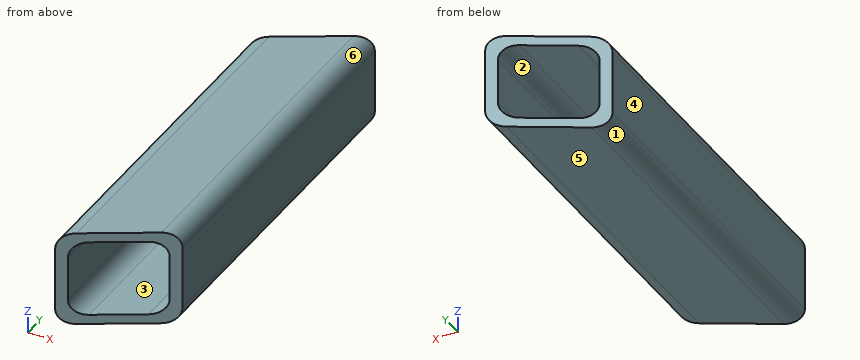
from build123d import *

# Parameters (mm, degrees)
F0_W     = 60
F0_H     = 60
F1_DEPTH = 250
F2_T     = -6
F3_R     = 10
F5_DEPTH = 60.001
F7_DEPTH = 60.001


with BuildPart() as f1:
    # F0 (on Front) → F1 (new body)
    with BuildSketch(Plane.XZ):
        Rectangle(F0_W, F0_H)
    extrude(amount=F1_DEPTH)

    # F2
    f2_openings = [f1.faces().sort_by_distance(p)[0] for p in [
        (0, -250, 0),
        (0, 0, 0),
    ]]
    offset(amount=F2_T, openings=f2_openings)

    # F3
    f3_edges = [f1.edges().sort_by_distance(p)[0] for p in [
        (-30, -125, 30),
        (-24, -125, -24),
        (30, -125, 30),
        (30, -125, -30),
        (-24, -125, 24),
        (-30, -125, -30),
        (24, -125, 24),
        (24, -125, -24),
    ]]
    fillet(f3_edges, radius=F3_R)

    # F4 (on face) → F5 (cut, through all)
    with BuildSketch(Plane.XY.offset(30)):
        Polygon((40, -255.7735026919), (40, -209.5854811567), (-40, -255.7735026919), align=None)
    extrude(amount=-F5_DEPTH, mode=Mode.SUBTRACT)

    # F6 (on face) → F7 (cut, through all)
    with BuildSketch(Plane.XY.offset(30)):
        Polygon((-40, 5.7735026919), (-40, -40.4145188433), (40, 5.7735026919), align=None)
    extrude(amount=-F7_DEPTH, mode=Mode.SUBTRACT)


solid = f1.part
CAD build for the part. Positions are in the model's coordinates, mm. Face numbers are marked on the shaded views. A direction names the side the tool comes from. Round coordinates to 2 decimals unless told otherwise and drop trailing zeros. Loops run counter-clockwise (first coordinate to the right, second up) from the corner with the lowest first, then second, coordinate; pieces in that order, holes last. Notation, with made-up numbers: M 81.5,2 L 137.5,2 A29 ccw 137.5,39 Z; hole C 3.5,2 d10. An arc over 180 degrees is marked long. One line per question, with ' | ' between items. Start each with the question number.
Item 1: Cut at A-A, the plane z = -2. Write the cut outline in (x, y).
Item 2: Wall check: line 1 (X direction, y = -112, z = 15); line 2 (X direction, y = -156, z = 1.5). Give the ranges that are in metal, low to high.
Item 3: Two-plate mould, pull along Z, no slides. Class the marked faces 3, 4, 5 and 6: pulls with the +Z half, pulls with the -Z half, needs draft (parallel to the pull), parting line crosses it, or undercut.
Item 4: Cut at C-C, the plane x = -5.5. Write the cut outline in (y, z), plus the area to 3 significant figures.
Item 5: Cut at B-B, the plane y = -166.5. Write the cut outline in (x, z).
Item 6: Which spindle directions (+Z, -Z, +X, -X, +Y, -Y) get a long thin tool onto all of the face, cutting with end or side? Do the marked faces 1 and 2. Say none if no direction does.
Item 7: Pin check, flat tip, straight feed: pin 1 Ø6 at (x, z) = (-21.5, 18) entering from -Y. Stop position of the tip, or through.
Responses:
1) outline: M -30,-250 L -24,-246.54 L -24,-31.18 L -30,-34.64 Z; M 24,-218.82 L 30,-215.36 L 30,0 L 24,-3.46 Z
2) line 1: x = -30 to -23.95, 23.95 to 30 | line 2: x = -30 to -24, 24 to 30
3) face 3: undercut | face 4: needs draft | face 5: pulls with the -Z half | face 6: pulls with the +Z half
4) outline: M -235.85,-30 L -20.5,-30 L -20.5,-24 L -235.85,-24 Z; M -235.85,24 L -20.5,24 L -20.5,30 L -235.85,30 Z | area: 2,580 mm²
5) outline: M -30,-20 A10 ccw -20,-30 L 20,-30 A10 ccw 30,-20 L 30,20 A10 ccw 20,30 L -20,30 A10 ccw -30,20 Z; hole M -24,-14 A10 ccw -14,-24 L 14,-24 A10 ccw 24,-14 L 24,14 A10 ccw 14,24 L -14,24 A10 ccw -24,14 Z
6) face 1: -Z, -X, +Y, -Y | face 2: +Y, -Y
7) pin 1: stops at y = -246.82
